Source: CAD feature listing. Evaluate the final solid. Frame: model axes, mm. Face numbers are marked on the shaded views. Round coordinates to 2 decimals unless told otherwise and drop trailing zeros. Write each loop counter-clockwise with the first axis right and the second up, starting at its lowest first coordinate (ties: lowest second). Pieces come first, ordered by that corner, then holes.
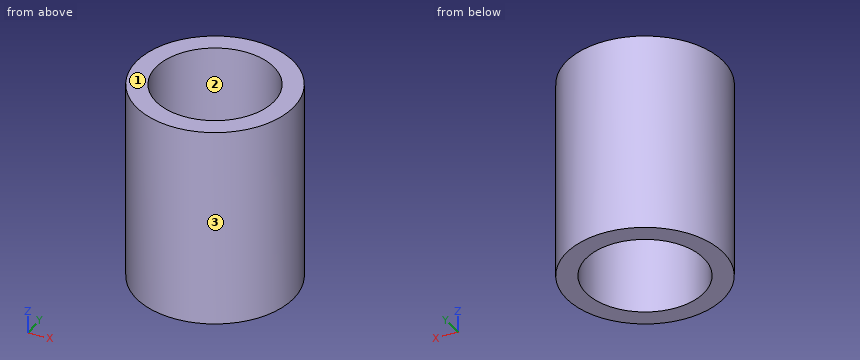
from build123d import *

# Parameters (mm, degrees)
CYLINDER_R        = 5.9
CYLINDER_DEPTH    = 20
CYLINDER001_R     = 7.85
CYLINDER001_DEPTH = 20


with BuildPart() as cylinder:
    # Cylinder → Cylinder (new body)
    with BuildSketch(Plane.XY):
        Circle(CYLINDER_R)
    extrude(amount=CYLINDER_DEPTH)


with BuildPart() as wheel_spacer:
    # Cylinder001 → Cylinder001 (new body)
    with BuildSketch(Plane.XY):
        Circle(CYLINDER001_R)
    extrude(amount=CYLINDER001_DEPTH)

    # Cut: cut Cylinder
    add(cylinder.part, mode=Mode.SUBTRACT)


solid = wheel_spacer.part
1) Contact query for flat-ended pins moving along their axis: P1, Ø1.5, axis at y = 5.5, z = 6.5, coming from the +X side; P2, Ø2, axis at x = -2.5, z = 7.5, coming from the -Y side; P3, Ø8, axis at y = 6, z = 13.5, coming from the +X side. Output: stop coordinate, or through.
Taken from the geometry:
P1: stops at x = 6.25
P2: stops at y = -7.71
P3: stops at x = 7.59
2) Section query D-D on y = -6.5. Return the cut outline in (x, z).
Taken from the geometry:
outline: (-4.4, 0) - (4.4, 0) - (4.4, 20) - (-4.4, 20) - close
3) Material intervals for line 1 (Y direction, x = 0, z = 7); line 2 (X direction, y = 0.25, z = 13.25); line 3 (Y direction, x = 3.5, z = 10), sorted ascending.
Taken from the geometry:
line 1: y = -7.85 to -5.9, 5.9 to 7.85
line 2: x = -7.85 to -5.89, 5.89 to 7.85
line 3: y = -7.03 to -4.75, 4.75 to 7.03
4) Section query A-A on y = 0. Return the cut outline in (x, z), then the cut area to 3 significant figures.
Taken from the geometry:
outline: (-7.85, 0) - (-5.9, 0) - (-5.9, 20) - (-7.85, 20) - close; (5.9, 0) - (7.85, 0) - (7.85, 20) - (5.9, 20) - close
area: 78.0 mm2
5) Pull-direction query (Y, two-part tool) for the marked faces 1, 2 and 3; classes: released by +Y, released by -Y, zero draft, split by the parting line, or undercut.
Taken from the geometry:
face 1: zero draft
face 2: undercut
face 3: split by the parting line
6) Section query C-C on z = 8.25. Return the cut outline in (x, y), then the cut area to 3 significant figures.
Taken from the geometry:
outline: circle Ø15.7 at (0, 0); hole circle Ø11.8 at (0, 0)
area: 84.2 mm2
